For this review, use the dimensioned drawing (mm, ordinates from the lowest corner) and the shaded views. A direction names the side the tool comes from. Round coordinates to 2 decimals unless told otherwise and drop trailing zeros. Loops run counter-clockwise (first coordinate to the right, second up) from the corner with the lowest first, then second, coordinate; pieces in that order, holes last. Notation, with made-up numbers: (-25.75, 43) -> (14.25, 43) arc R18 cw to (14.25, 52) -> close; hole circle Ø3 at (73.25, 36). An arc over 180 degrees is marked (long way). Answer as CSV lines item,"result". Start each with the question number.
(1) Take a section at D-D, the plane z = 0.45. Write out the cut boundary in (x, y) (3 decimals), and give its area (3 significant figures).
(2) Take a section at C-C, the plane y = 2.5. Write out the cut boundary in (x, z).
(3) Take a section at B-B, the plane x = 2.5. Write out the cut boundary in (y, z).
(4) Take a section at A-A, the plane y = 4.5. Write out the cut boundary in (x, z), and give its area (3 significant figures).
(5) For P1, Ø2.5, axis at x = 2.5, y = 15, coming from the +Z side, flat-tipped, find the tip position at first contact; note if it passes through.
(6) Draft analysis for pull direction X (two halves, no side actions). For the marked faces 1, 2, 3 and 4, state which applies: +X half, -X half, draft (parallel to the pull), parting line (faces both ways), or undercut.
(7) To check wall thickness, follow line 1 (X direction, y = 2.5, z = 0.4); line 2 (X direction, y = 14.5, z = 0.9); line 3 (X direction, y = 13, z = 0.2). State the ranges of each line that lie inside material, in increasing order. Write a range as from..to.
(8) Machinability: for the marked faces 5, 6 and 7, which of the approach directions +Z, -Z, +X, -X, +Y, -Y give a long, thin tool a straight path to every point of the face, cutting with its end or side? Answer none if there is none.
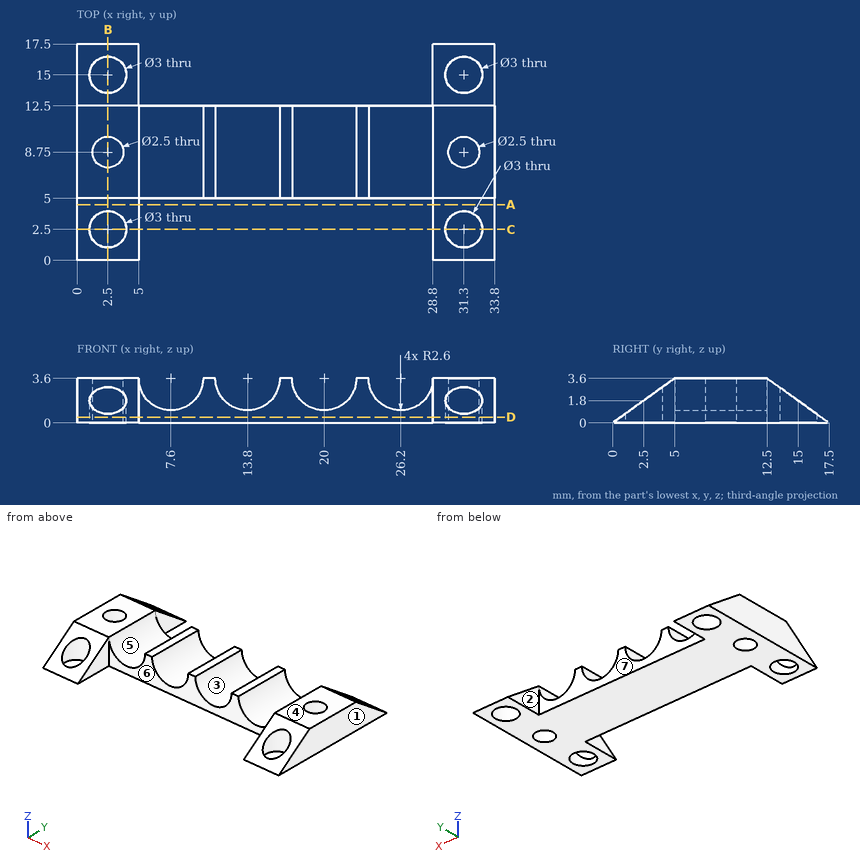
The answers:
1,outline,"(0, 0.625) -> (5, 0.625) -> (5, 5) -> (28.8, 5) -> (28.8, 0.625) -> (33.8, 0.625) -> (33.8, 16.875) -> (28.8, 16.875) -> (28.8, 12.5) -> (5, 12.5) -> (5, 16.875) -> (0, 16.875) -> close; hole circle Ø3 at (2.5, 2.5); hole circle Ø3 at (2.5, 15); hole circle Ø2.5 at (2.5, 8.75); hole circle Ø3 at (31.3, 2.5); hole circle Ø3 at (31.3, 15); hole circle Ø2.5 at (31.3, 8.75)"
1,area,"303 mm²"
2,outline,"(0, 0) -> (1, 0) -> (1, 1.8) -> (0, 1.8) -> close; (4, 0) -> (5, 0) -> (5, 1.8) -> (4, 1.8) -> close; (28.8, 0) -> (29.8, 0) -> (29.8, 1.8) -> (28.8, 1.8) -> close; (32.8, 0) -> (33.8, 0) -> (33.8, 1.8) -> (32.8, 1.8) -> close"
3,outline,"(0, 0) -> (1, 0) -> (1, 0.72) -> close; (4, 0) -> (7.5, 0) -> (7.5, 3.6) -> (5, 3.6) -> (4, 2.88) -> close; (10, 0) -> (13.5, 0) -> (13.5, 2.88) -> (12.5, 3.6) -> (10, 3.6) -> close; (16.5, 0) -> (17.5, 0) -> (16.5, 0.72) -> close"
4,outline,"(0, 0) -> (5, 0) -> (5, 3.24) -> (0, 3.24) -> close; (28.8, 0) -> (33.8, 0) -> (33.8, 3.24) -> (28.8, 3.24) -> close"
4,area,"32.4 mm²"
5,P1,"through"
6,face 1,"+X half"
6,face 2,"undercut"
6,face 3,"undercut"
6,face 4,"draft"
7,line 1,"0..1, 4..5, 28.8..29.8, 32.8..33.8"
7,line 2,"0..1.09, 3.91..5, 28.8..29.89, 32.71..33.8"
7,line 3,"0..5, 28.8..33.8"
8,face 5,"+Z, +Y, -Y"
8,face 6,"+Z, -Z, -Y"
8,face 7,"+Z, -Z, +Y"
